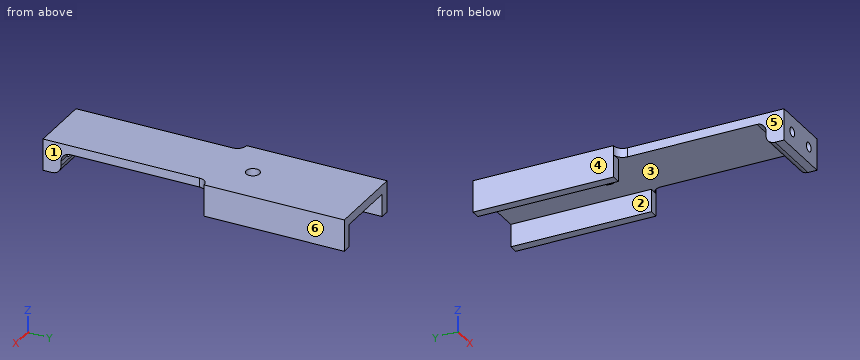
```python
from build123d import *

# Parameters (mm, degrees)
SKETCH2_W                       = 14
SKETCH2_H                       = 31
SKETCH2_R                       = 1.5
SKETCH2_H_2                     = 36.9
BOSS_EXTRUDE1_DEPTH             = 2
SKETCH3_W                       = 14
SKETCH3_H                       = 4
BOSS_EXTRUDE2_DEPTH             = 5
SKETCH4_R                       = 1
CUT_EXTRUDE1_DEPTH              = 4
SKETCH5_W                       = 0.075
SKETCH5_H                       = 31
SKETCH5_H_2                     = 0.15
BOSS_EXTRUDE3_DEPTH             = 5
BOSS_EXTRUDE3_DIRECTION_2_REACH = 55.101
FILLET1_R                       = 2


with BuildPart() as part:
    # Sketch2 → Boss-Extrude1 (new body)
    # profile 1 of 3: a face of its own
    with BuildSketch(Plane.XY):
        Rectangle(SKETCH2_W, SKETCH2_H)
        with BuildLine():
            ThreePointArc((1.7, -9.5), (0, -11.2), (-1.7, -9.5))
            ThreePointArc((-1.7, -9.5), (0, -7.8), (1.7, -9.5))
        make_face(mode=Mode.SUBTRACT)
    # profile 2 of 3: a face of its own
    with BuildSketch(Plane.XY):
        with BuildLine():
            ThreePointArc((-1.7, -9.5), (0, -7.8), (1.7, -9.5))
            ThreePointArc((1.7, -9.5), (0, -11.2), (-1.7, -9.5))
        make_face()
        with Locations((0, -9.5)):
            Circle(SKETCH2_R, mode=Mode.SUBTRACT)
    # profile 3 of 3: a face of its own
    with BuildSketch(Plane.XY):
        with Locations((0, -33.95)):
            Rectangle(SKETCH2_W, SKETCH2_H_2)
    extrude(amount=BOSS_EXTRUDE1_DEPTH)

    # Sketch3 → Boss-Extrude2 (add)
    with BuildSketch(Plane(origin=(0, 0, 0), x_dir=(-1, 0, 0), z_dir=(0, 0, -1))):
        with Locations((0, -50.4)):
            Rectangle(SKETCH3_W, SKETCH3_H)
    extrude(amount=BOSS_EXTRUDE2_DEPTH)

    # Sketch4 → Cut-Extrude1 (cut)
    with BuildSketch(Plane.XZ.offset(52.4)):
        with Locations(Location((-3.5, -1.5, 0), (0, 0, 270))):
            Circle(SKETCH4_R)
        with Locations(Location((3.5, -1.5, 0), (0, 0, 270))):
            Circle(SKETCH4_R)
    extrude(amount=-CUT_EXTRUDE1_DEPTH, mode=Mode.SUBTRACT)

    # Sketch5 → Boss-Extrude3 (add)
    with BuildSketch(Plane(origin=(0, 0, 0), x_dir=(-1, 0, 0), z_dir=(0, 0, -1))):
        Polygon((-7.075, -15.65), (-7.075, -15.5), (-7.075, 15.5), (-9.075, 15.5), (-9.075, -15.65), align=None)
        Polygon((7.075, 15.5), (7.075, -15.5), (7.075, -15.65), (9.075, -15.65), (9.075, 15.5), align=None)
        with Locations((7.0375, 0)):
            Rectangle(SKETCH5_W, SKETCH5_H)
        with Locations((-7.0375, 0)):
            Rectangle(SKETCH5_W, SKETCH5_H)
        with Locations((-7.0375, -15.575)):
            Rectangle(SKETCH5_W, SKETCH5_H_2)
        with Locations((7.0375, -15.575)):
            Rectangle(SKETCH5_W, SKETCH5_H_2)
    extrude(amount=BOSS_EXTRUDE3_DEPTH)

    # Boss-Extrude3 direction 2: up to this face of the body (flat: up to its plane)
    boss_extrude3_direction_2_end = Plane(part.part.faces().sort_by_distance((0, -18.517050043, 2))[0])
    # Sketch5 → Boss-Extrude3 direction 2 (add, up to the picked face)
    with BuildSketch(Plane(origin=(0, 0, 0), x_dir=(-1, 0, 0), z_dir=(0, 0, -1)), mode=Mode.PRIVATE) as boss_extrude3_direction_2_sk1:
        Polygon((-7.075, -15.65), (-7.075, -15.5), (-7.075, 15.5), (-9.075, 15.5), (-9.075, -15.65), align=None)
    boss_extrude3_direction_2_tool1 = split(extrude(boss_extrude3_direction_2_sk1.sketch, amount=-BOSS_EXTRUDE3_DIRECTION_2_REACH, mode=Mode.PRIVATE), bisect_by=boss_extrude3_direction_2_end, keep=Keep.BOTH, mode=Mode.PRIVATE)
    # Sketch5 → Boss-Extrude3 direction 2 (add, up to the picked face)
    with BuildSketch(Plane(origin=(0, 0, 0), x_dir=(-1, 0, 0), z_dir=(0, 0, -1)), mode=Mode.PRIVATE) as boss_extrude3_direction_2_sk2:
        Polygon((7.075, 15.5), (7.075, -15.5), (7.075, -15.65), (9.075, -15.65), (9.075, 15.5), align=None)
    boss_extrude3_direction_2_tool2 = split(extrude(boss_extrude3_direction_2_sk2.sketch, amount=-BOSS_EXTRUDE3_DIRECTION_2_REACH, mode=Mode.PRIVATE), bisect_by=boss_extrude3_direction_2_end, keep=Keep.BOTH, mode=Mode.PRIVATE)
    # Sketch5 → Boss-Extrude3 direction 2 (add, up to the picked face)
    with BuildSketch(Plane(origin=(0, 0, 0), x_dir=(-1, 0, 0), z_dir=(0, 0, -1)), mode=Mode.PRIVATE) as boss_extrude3_direction_2_sk3:
        with Locations((7.0375, 0)):
            Rectangle(SKETCH5_W, SKETCH5_H)
    boss_extrude3_direction_2_tool3 = split(extrude(boss_extrude3_direction_2_sk3.sketch, amount=-BOSS_EXTRUDE3_DIRECTION_2_REACH, mode=Mode.PRIVATE), bisect_by=boss_extrude3_direction_2_end, keep=Keep.BOTH, mode=Mode.PRIVATE)
    # Sketch5 → Boss-Extrude3 direction 2 (add, up to the picked face)
    with BuildSketch(Plane(origin=(0, 0, 0), x_dir=(-1, 0, 0), z_dir=(0, 0, -1)), mode=Mode.PRIVATE) as boss_extrude3_direction_2_sk4:
        with Locations((-7.0375, 0)):
            Rectangle(SKETCH5_W, SKETCH5_H)
    boss_extrude3_direction_2_tool4 = split(extrude(boss_extrude3_direction_2_sk4.sketch, amount=-BOSS_EXTRUDE3_DIRECTION_2_REACH, mode=Mode.PRIVATE), bisect_by=boss_extrude3_direction_2_end, keep=Keep.BOTH, mode=Mode.PRIVATE)
    # Sketch5 → Boss-Extrude3 direction 2 (add, up to the picked face)
    with BuildSketch(Plane(origin=(0, 0, 0), x_dir=(-1, 0, 0), z_dir=(0, 0, -1)), mode=Mode.PRIVATE) as boss_extrude3_direction_2_sk5:
        with Locations((-7.0375, -15.575)):
            Rectangle(SKETCH5_W, SKETCH5_H_2)
    boss_extrude3_direction_2_tool5 = split(extrude(boss_extrude3_direction_2_sk5.sketch, amount=-BOSS_EXTRUDE3_DIRECTION_2_REACH, mode=Mode.PRIVATE), bisect_by=boss_extrude3_direction_2_end, keep=Keep.BOTH, mode=Mode.PRIVATE)
    # Sketch5 → Boss-Extrude3 direction 2 (add, up to the picked face)
    with BuildSketch(Plane(origin=(0, 0, 0), x_dir=(-1, 0, 0), z_dir=(0, 0, -1)), mode=Mode.PRIVATE) as boss_extrude3_direction_2_sk6:
        with Locations((7.0375, -15.575)):
            Rectangle(SKETCH5_W, SKETCH5_H_2)
    boss_extrude3_direction_2_tool6 = split(extrude(boss_extrude3_direction_2_sk6.sketch, amount=-BOSS_EXTRUDE3_DIRECTION_2_REACH, mode=Mode.PRIVATE), bisect_by=boss_extrude3_direction_2_end, keep=Keep.BOTH, mode=Mode.PRIVATE)
    add(boss_extrude3_direction_2_tool1.solids().sort_by(Axis((8.075, -0.075, 0), (0, 0, 1)))[0])
    add(boss_extrude3_direction_2_tool2.solids().sort_by(Axis((-8.075, -0.075, 0), (0, 0, 1)))[0])
    add(boss_extrude3_direction_2_tool3.solids().sort_by(Axis((-7.0375, 0, 0), (0, 0, 1)))[0])
    add(boss_extrude3_direction_2_tool4.solids().sort_by(Axis((7.0375, 0, 0), (0, 0, 1)))[0])
    add(boss_extrude3_direction_2_tool5.solids().sort_by(Axis((7.0375, -15.575, 0), (0, 0, 1)))[0])
    add(boss_extrude3_direction_2_tool6.solids().sort_by(Axis((-7.0375, -15.575, 0), (0, 0, 1)))[0])

    # Fillet1
    # the kernel refuses this fillet: 2 mm, written as the material it adds along each edge
    with BuildSketch(Plane(origin=(7, -48.4, 0), x_dir=(0, 0, -1), z_dir=(-1, 0, 0))) as fillet1_piece_1_section:
        with BuildLine():
            CenterArc((FILLET1_R, -FILLET1_R), FILLET1_R, 90, 90)
            Line((0, -FILLET1_R), (0, 0))
            Line((0, 0), (FILLET1_R, 0))
        make_face()
    fillet1_piece_1 = extrude(amount=14, mode=Mode.PRIVATE)
    fillet1_piece_1 = fillet1_piece_1 - Plane(origin=(-3.5, -47.93211331, -1.5), x_dir=(0, 0, -1), z_dir=(0, -1, 0)) * Cylinder(1, 37, mode=Mode.PRIVATE)
    fillet1_piece_1 = fillet1_piece_1 - Plane(origin=(3.5, -47.93211331, -1.5), x_dir=(0, 0, -1), z_dir=(0, -1, 0)) * Cylinder(1, 37, mode=Mode.PRIVATE)
    add(fillet1_piece_1)
    with BuildSketch(Plane(origin=(7, -15.65, 0), x_dir=(0, -1, 0), z_dir=(0, 0, 1)), Plane(origin=(-7, -15.65, 0), x_dir=(-1, 0, 0), z_dir=(0, 0, 1))) as fillet1_piece_2:
        with BuildLine():
            CenterArc((FILLET1_R, FILLET1_R), FILLET1_R, 180, 90)
            Line((0, FILLET1_R), (0, 0))
            Line((0, 0), (FILLET1_R, 0))
        make_face()
    extrude(amount=2)
    # the kernel refuses this fillet: 2 mm, written as the material it takes off along each edge
    with BuildSketch(Plane(origin=(12, -48.4, -5), x_dir=(0, 0, 1), z_dir=(-1, 0, 0))) as fillet1_2_piece_1:
        with BuildLine():
            CenterArc((FILLET1_R, -FILLET1_R), FILLET1_R, 90, 90)
            Line((0, -FILLET1_R), (0, 0))
            Line((0, 0), (FILLET1_R, 0))
        make_face()
    extrude(amount=24, mode=Mode.SUBTRACT)


solid = part.part
```
CAD build for the part. Positions are in the model's coordinates, mm. Face numbers are marked on the shaded views. A direction names the side the tool comes from. Give positions to 0.01 mm unless a question says otherwise; leave off trailing zeros. Loops run counter-clockwise (first coordinate to the right, second up) from the corner with the lowest first, then second, coordinate; pieces in that order, holes last. Notation, with made-up numbers: (27, 38) -> (85, 38) arc R6 cw to (85, 48) -> close; hole circle Ø4 at (-12, 54). An arc over 180 degrees is marked (long way). Use a Markdown table: item, result.
1. Slice it at A-A (x = 0). List the corners of the cut face in (y, z), plus the area to 3 significant figures.
Check result:
| item | result |
|---|---|
| outline | (-52.4, -5) -> (-50.4, -5) arc R2 ccw to (-48.4, -3) -> (-48.4, -2) arc R2 cw to (-46.4, 0) -> (-11, 0) -> (-11, 2) -> (-52.4, 2) -> close; (-8, 0) -> (15.5, 0) -> (15.5, 2) -> (-8, 2) -> close |
| area | 150 mm^2 |
2. Wall check: L1, parallel to X at y = -50.3, z = -1.5; L2, parallel to X at y = 4, z = -0.75 (3 decimals); L3, parallel to Z at x = 1.75, y = -36. Give the ranges that are in metal, low to high. Write a range as [from, to].
Check result:
| item | result |
|---|---|
| L1 | x = [-7, -4.5], [-2.5, 2.5], [4.5, 7] |
| L2 | x = [-9.075, -7], [7, 9.075] |
| L3 | z = [0, 2] |
3. Slice it at B-B (y = -9.5). List the corners of the cut face in (x, z) (3 decimals), plus the area to 4 significant figures.
Check result:
| item | result |
|---|---|
| outline | (-9.075, -5) -> (-7, -5) -> (-7, 0) -> (-1.5, 0) -> (-1.5, 2) -> (-9.075, 2) -> close; (1.5, 0) -> (7, 0) -> (7, -5) -> (9.075, -5) -> (9.075, 2) -> (1.5, 2) -> close |
| area | 51.05 mm^2 |
4. Flat gauge pins, fed straight in: pin 1 (1 mm diameter, centred on x = 8, z = -2, fed in from -Y); pin 2 (1.8 mm diameter, centred on x = 0, y = -9.5, fed in from -Z); pin 3 (5.5 mm diameter, centred on x = 4, y = -29, fed in from -Z); pin 4 (4 mm diameter, centred on y = -34, z = 0, fed in from -X). Where does each tip first touch, or does it go through?
Check result:
| item | result |
|---|---|
| pin 1 | stops at y = -15.65 |
| pin 2 | passes through |
| pin 3 | stops at z = 0 |
| pin 4 | stops at x = -7 |
5. Slice it at D-D (y = 2). List the corners of the cut face in (x, z) (3 decimals).
Check result:
| item | result |
|---|---|
| outline | (-9.075, -5) -> (-7, -5) -> (-7, 0) -> (7, 0) -> (7, -5) -> (9.075, -5) -> (9.075, 2) -> (-9.075, 2) -> close |
6. Mould opens along X. For the marked faces 1, 2, 3 and 4 say: pulls with the +X half, pulls with the -X half, needs draft (parallel to the pull), parting line crosses it, or undercut.
Check result:
| item | result |
|---|---|
| face 1 | pulls with the +X half |
| face 2 | undercut |
| face 3 | undercut |
| face 4 | pulls with the -X half |
7. Slice it at C-C (z = -4). List the corners of the cut face in (x, y) (3 decimals).
Check result:
| item | result |
|---|---|
| outline | (-9.075, -15.65) -> (-7, -15.65) -> (-7, 15.5) -> (-9.075, 15.5) -> close; (-7, -52.4) -> (7, -52.4) -> (7, -48.668) -> (-7, -48.668) -> close; (7, -15.65) -> (9.075, -15.65) -> (9.075, 15.5) -> (7, 15.5) -> close |
8. Which spindle directions (+Z, -Z, +X, -X, +Y, -Y) get a long thin tool onto all of the face, cutting with end or side? Do the marked faces 5 and 6. Say none if no direction does.
Check result:
| item | result |
|---|---|
| face 5 | +Z, -Z, -X, -Y |
| face 6 | +Z, -Z, +X, +Y, -Y |
